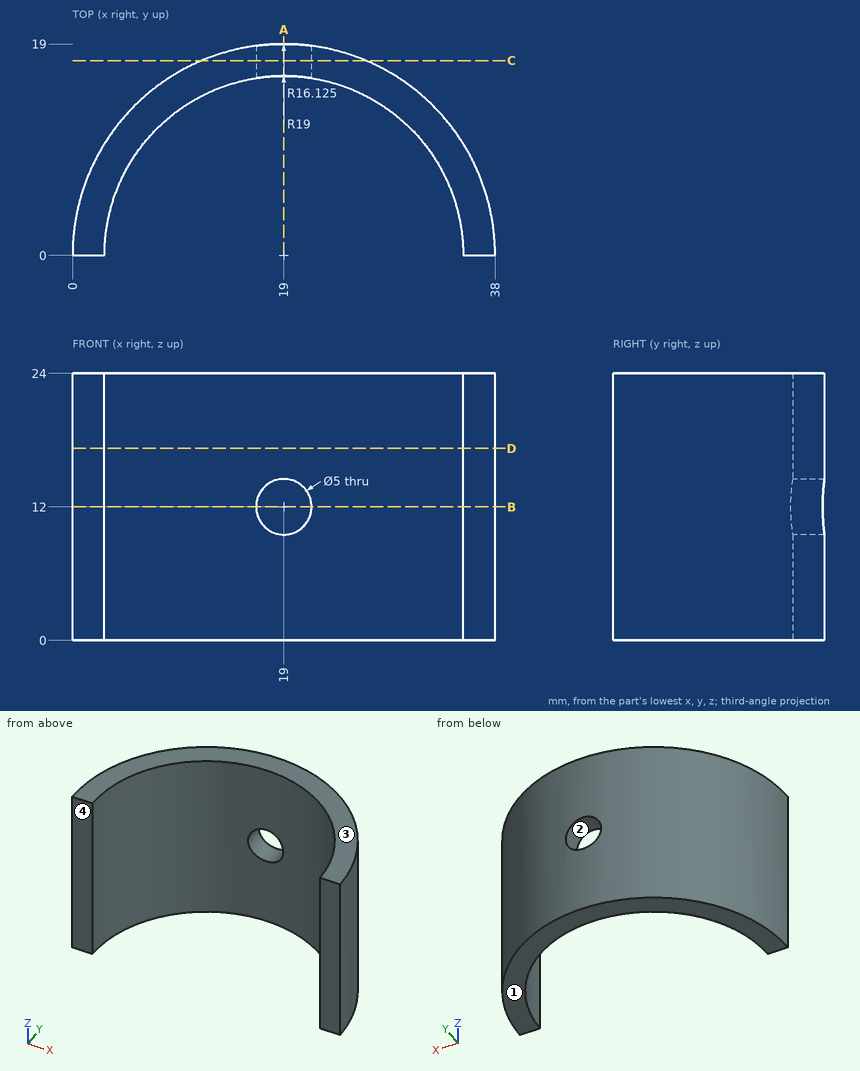
Here's the drawing with two shaded views (mm, measured from the low corner). I have some questions. Round coordinates to 2 decimals unless told otherwise and drop trailing zeros. Write each loop counter-clockwise with the first axis right and the second up, starting at its lowest first coordinate (ties: lowest second). Pieces come first, ordered by that corner, then holes. Notation, with made-up numbers: M 53,-22.5 L 58,-22.5 A16 ccw 58,-11.5 Z; hole C 40,54.5 d5. An arc over 180 degrees is marked long. Use CSV: the item, a comma, the result in double quotes.
(1) Imagine slicing it at B-B (z = 12). Write out the boundary of the cut face in (x, y) (3 decimals).
Check values:
outline,"M 0,0 L 2.875,0 A16.125 cw 16.5,15.93 L 16.5,18.835 A19 ccw Z; M 21.5,15.93 A16.125 cw 35.125,0 L 38,0 A19 ccw 21.5,18.835 Z"
(2) We'd pull the mould along Z, two halves only. Please class the marked faces 1, 2, 3 and 4: +Z half, -Z half, draft (parallel to the pull), parting line (faces both ways), or undercut.
Check values:
face 1,"-Z half"
face 2,"undercut"
face 3,"+Z half"
face 4,"draft"
(3) Imagine slicing it at C-C (y = 17.5). Write out the boundary of the cut face in (x, z), plus the area to 3 significant figures.
Check values:
outline,"M 11.6,0 L 26.4,0 L 26.4,24 L 11.6,24 Z; hole C 19,12 d5"
area,"336 mm^2"
(4) I'm going to push flat-ended pins straight in: pin 1 (6 mm diameter, centred on x = 30, z = 7.5, fed in from -Y); pin 2 (1 mm diameter, centred on y = 7, z = 3.5, fed in from -X); pin 3 (8 mm diameter, centred on y = 8, z = 5.5, fed in from +X). Where does each tip first touch, or does it pass through?
Check values:
pin 1,"y = 8"
pin 2,"x = 1.15"
pin 3,"x = 37.57"
(5) I need wall thicknesses on line 1 along Z through (x, y) = (19, 17.55); line 2 along X through (y, z) = (10.5, 2.75); line 3 along X through (y, z) = (1.5, 3). Which ranges of each line are inside material? Lowest first, please.
Check values:
line 1,"0 to 9.5, 14.5 to 24"
line 2,"3.16 to 6.76, 31.24 to 34.84"
line 3,"0.06 to 2.94, 35.06 to 37.94"
(6) Imagine slicing it at A-A (x = 19). Write out the boundary of the cut face in (y, z) (3 decimals), plus the area to 3 significant figures.
Check values:
outline,"M 16.125,0 L 19,0 L 19,9.5 L 16.125,9.5 Z; M 16.125,14.5 L 19,14.5 L 19,24 L 16.125,24 Z"
area,"54.6 mm^2"
(7) Imagine slicing it at D-D (z = 17.25). Write out the boundary of the cut face in (x, y) (3 decimals).
Check values:
outline,"M 0,0 L 2.875,0 A16.125 cw 35.125,0 L 38,0 A19 ccw Z"
